Here's how the part is built. I have some questions about the finished solid (model axes, mm). A direction names the side the tool comes from. Give positions to 0.01 mm unless a question says otherwise; leave off trailing zeros. Write each loop counter-clockwise with the first axis right and the second up, starting at its lowest first coordinate (ties: lowest second). Pieces come first, ordered by that corner, then holes. Notation, with made-up numbers: (9.25, -1.75) -> (30.25, -1.75) arc R21 ccw to (30.25, 28.25) -> close; hole circle Ø2 at (56.5, 63). An arc over 180 degrees is marked (long way). Put each result on its own line as item: value. Start each with the question number.
from build123d import *

# Parameters (mm, degrees)
CHAMFER1_SIZE = 1


with BuildPart() as part:
    # Sketch1 → Revolve1 (revolve)
    with BuildSketch(Plane.XY, mode=Mode.PRIVATE) as revolve1_sk:
        Polygon((1.75, 0), (7.9, 0), (7.9, 7.5), (9.9, 7.5), (9.9, 8.5), (3.5, 8.5), (3.5, 5.5), (3, 5.5), (3, 5), (1.75, 5), align=None)
    revolve(revolve1_sk.sketch.rotate(Axis((0, 37.275, 0), (0, -1, 0)), 90), axis=Axis((0, 37.275, 0), (0, -1, 0)))

    # Chamfer1
    chamfer1_edges = [part.edges().sort_by_distance(p)[0] for p in [
        (0, 0, -7.9),
    ]]
    chamfer(chamfer1_edges, length=CHAMFER1_SIZE)


solid = part.part
1) I want a section at B-B, the plane x = 0. Write out the boundary of the cut face in (y, z), and give its area (3 significant figures).
2) I want a section at D-D, the plane y = 7.25. Write out the boundary of the cut face in (x, z).
3) I'm going to push flat-ended pins straight in: pin 1 Ø4 at (y, z) = (2, 4.5) entering from -X; pin 2 Ø1.8 at (x, z) = (-0.5, 1.5) entering from +Y; pin 3 Ø1.5 at (y, z) = (3.5, -0.5) entering from -X. Where does each tip first touch, or does it pass through?
4) Which directions (+Z, -Z, +X, -X, +Y, -Y) give clear straight access to the entire face, cutting with the end or side of a thin tool? Please do faces 5 (the flat face through (-1, 5.5, 3)), 6 (the cylindrical face through (-5.34, 4.3, -5.82)), 7 (the flat face through (4, 8.5, 0)).
5) I want a section at A-A, the plane z = 0. Write out the boundary of the cut face in (x, y).
6) I want a section at C-C, the plane y = 3. Write out the boundary of the cut face in (x, z).
7) Thinking about a two-plate mould opening in X: for faces 1 (the cylindrical face through (-2.974, 8.007, 9.443)), 2 (the flat face through (2, 5, 0)), 3 (the cylindrical face through (-0.9, 5.25, 2.86)), 4 (the flat face through (1.4, 0, -1.4)), which applies, released by +X, released by -X, zero draft, split by the parting line, or undercut?
8) I need wall thicknesses on probe 1 along X at (y, z) = (7.6, 0); probe 2 along X at (y, z) = (6.5, 0); probe 3 along Y at (x, z) = (-8.5, 1.75). Which ranges of each line are inside material? Lowest first, please.
Established:
1. outline: (0, -6.9) -> (1, -7.9) -> (7.5, -7.9) -> (7.5, -9.9) -> (8.5, -9.9) -> (8.5, -3.5) -> (5.5, -3.5) -> (5.5, -3) -> (5, -3) -> (5, -1.75) -> (0, -1.75) -> close; (0, 1.75) -> (5, 1.75) -> (5, 3) -> (5.5, 3) -> (5.5, 3.5) -> (8.5, 3.5) -> (8.5, 9.9) -> (7.5, 9.9) -> (7.5, 7.9) -> (1, 7.9) -> (0, 6.9) -> close
1. area: 95.8 mm2
2. outline: circle Ø15.8 at (0, 0); hole circle Ø7 at (0, 0)
3. pin 1: stops at x = -7.49
3. pin 2: stops at y = 5
3. pin 3: stops at x = -7.9
4. face 5: +Y
4. face 6: -Y
4. face 7: +Z, -Z, +X, -X, +Y
5. outline: (-9.9, 7.5) -> (-7.9, 7.5) -> (-7.9, 1) -> (-6.9, 0) -> (-1.75, 0) -> (-1.75, 5) -> (-3, 5) -> (-3, 5.5) -> (-3.5, 5.5) -> (-3.5, 8.5) -> (-9.9, 8.5) -> close; (1.75, 0) -> (6.9, 0) -> (7.9, 1) -> (7.9, 7.5) -> (9.9, 7.5) -> (9.9, 8.5) -> (3.5, 8.5) -> (3.5, 5.5) -> (3, 5.5) -> (3, 5) -> (1.75, 5) -> close
6. outline: circle Ø15.8 at (0, 0); hole circle Ø3.5 at (0, 0)
7. face 1: split by the parting line
7. face 2: undercut
7. face 3: undercut
7. face 4: zero draft
8. probe 1: x = -9.9 to -3.5, 3.5 to 9.9
8. probe 2: x = -7.9 to -3.5, 3.5 to 7.9
8. probe 3: y = 7.5 to 8.5
